Here's how the part is built. I have some questions about the finished solid (model axes, mm). Face numbers are marked on the shaded views. Round coordinates to 2 decimals unless told otherwise and drop trailing zeros. Order: outer loops, then holes, each group sorted by start corner. A loop starts at its lowest first (then second) coordinate and runs counter-clockwise, first axis right, second up.
```python
from build123d import *

# Parameters (mm, degrees)
SKETCH1_W           = 15.24
SKETCH1_H           = 15.24
BOSS_EXTRUDE1_DEPTH = 1.5
SKETCH2_R           = 1.905
SKETCH2_R_2         = 0.635
CUT_EXTRUDE1_DEPTH  = 11.880202204
SKETCH3_W           = 3.95
SKETCH3_H           = 3.95
BOSS_EXTRUDE2_DEPTH = 0.75
BOSS_EXTRUDE3_DEPTH = 0.25


with BuildPart() as part:
    # Sketch1 → Boss-Extrude1 (new body)
    with BuildSketch(Plane(origin=(0, 0, 0), x_dir=(1, 0, 0), z_dir=(0, 1, 0))):
        Rectangle(SKETCH1_W, SKETCH1_H)
    extrude(amount=BOSS_EXTRUDE1_DEPTH)

    # Sketch2 → Cut-Extrude1 (cut, through all)
    with BuildSketch(Plane(origin=(0, 1.5, 0), x_dir=(1, 0, 0), z_dir=(0, 1, 0))):
        with Locations(Location((-5.08, 5.08, 0), (0, 0, 270))):
            Circle(SKETCH2_R)
        with Locations(Location((5.08, 5.08, 0), (0, 0, 270))):
            Circle(SKETCH2_R)
        with Locations(Location((5.08, -6.35, 0), (0, 0, 270))):
            Circle(SKETCH2_R_2)
        with Locations(Location((2.54, -6.35, 0), (0, 0, 270))):
            Circle(SKETCH2_R_2)
        with Locations(Location((0, -6.35, 0), (0, 0, 270))):
            Circle(SKETCH2_R_2)
        with Locations(Location((-2.54, -6.35, 0), (0, 0, 270))):
            Circle(SKETCH2_R_2)
        with Locations(Location((-5.08, -6.35, 0), (0, 0, 270))):
            Circle(SKETCH2_R_2)
    extrude(amount=-CUT_EXTRUDE1_DEPTH, mode=Mode.SUBTRACT)

    # Sketch3 → Boss-Extrude2 (add)
    with BuildSketch(Plane(origin=(0, 1.5, 0), x_dir=(1, 0, 0), z_dir=(0, 1, 0))):
        Rectangle(SKETCH3_W, SKETCH3_H)
    extrude(amount=BOSS_EXTRUDE2_DEPTH)

    # Sketch4 → Boss-Extrude3 (add)
    with BuildSketch(Plane(origin=(0, 2.25, 0), x_dir=(1, 0, 0), z_dir=(0, 1, 0))):
        with BuildLine():
            Line((-1.295144256, 1.380499313), (-1.087590503, 1.380499313))
            add(Edge.make_bspline(
                [(-1.087590503, 1.380499313), (-1.073314825, 1.38048362), (-1.04596199, 1.380453553), (-1.006738628, 1.379541951), (-0.971115209, 1.378324356), (-0.939168546, 1.376636498), (-0.910800345, 1.374641815), (-0.886138971, 1.371844174), (-0.864990582, 1.368923085), (-0.85231887, 1.365953279), (-0.846539822, 1.364598872)],
                knots=[0, 0, 0, 0, 1.415646017, 2.712440637, 3.8905458, 4.950247383, 5.884950622, 6.709939814, 7.411656543, 8, 8, 8, 8], degree=3))
            add(Edge.make_bspline(
                [(-0.846539822, 1.364598872), (-0.839224159, 1.362596521), (-0.824765215, 1.358639001), (-0.803930852, 1.35071247), (-0.784108618, 1.341313815), (-0.765230504, 1.33060229), (-0.747528493, 1.318118322), (-0.730738476, 1.304367966), (-0.715008625, 1.289033754), (-0.700427395, 1.272287673), (-0.687036515, 1.254410848), (-0.675506825, 1.235136412), (-0.66585264, 1.214788803), (-0.65757246, 1.193382176), (-0.651612999, 1.170736768), (-0.64712358, 1.147009929), (-0.644274054, 1.122204201), (-0.644001137, 1.105252765), (-0.643862205, 1.096623445)],
                knots=[0, 0, 0, 0, 0.999701418, 1.975846123, 2.934577507, 3.890451536, 4.834027766, 5.787354733, 6.749476667, 7.726910423, 8.712836071, 9.690891519, 10.682875813, 11.679750201, 12.712814741, 13.765529915, 14.8625177, 16, 16, 16, 16], degree=3))
            add(Edge.make_bspline(
                [(-0.643862205, 1.096623445), (-0.643989636, 1.087921593), (-0.644238963, 1.070895833), (-0.647231411, 1.045987871), (-0.651262207, 1.022184929), (-0.657460125, 0.999539786), (-0.665577745, 0.978186922), (-0.675100342, 0.957800025), (-0.686585838, 0.938725934), (-0.699783203, 0.920895401), (-0.714464281, 0.904291689), (-0.730566955, 0.889035121), (-0.748026217, 0.875214999), (-0.766786581, 0.862800343), (-0.78703094, 0.852079039), (-0.808452258, 0.842476235), (-0.831236728, 0.834411414), (-0.847003631, 0.830168991), (-0.855020057, 0.828012)],
                knots=[0, 0, 0, 0, 1.121902311, 2.195077645, 3.232258892, 4.234102512, 5.217864754, 6.176164875, 7.132989551, 8.084763148, 9.034132444, 9.988522005, 10.94243251, 11.903244335, 12.886203696, 13.894208494, 14.929344452, 16, 16, 16, 16], degree=3))
            add(Edge.make_bspline(
                [(-0.855020057, 0.828012), (-0.861650466, 0.826602003), (-0.87618139, 0.823511913), (-0.900112642, 0.820062213), (-0.927975652, 0.817117748), (-0.959732389, 0.814910024), (-0.995354348, 0.813020031), (-1.0348608, 0.811517774), (-1.078329294, 0.810692318), (-1.108649409, 0.810649745), (-1.124479526, 0.810627518)],
                knots=[0, 0, 0, 0, 0.601384939, 1.31797006, 2.144135048, 3.087295005, 4.142315834, 5.309527816, 6.595305764, 8, 8, 8, 8], degree=3))
            Line((-1.124479526, 0.810627518), (-1.200165624, 0.810627518))
            Line((-1.200165624, 0.810627518), (-1.200165624, 0.322165979))
            Line((-1.200165624, 0.322165979), (-1.295144256, 0.322165979))
            Line((-1.295144256, 0.322165979), (-1.295144256, 1.380499313))
        make_face()
        with BuildLine():
            Line((-1.200165624, 1.271952304), (-1.200165624, 0.919174527))
            Line((-1.200165624, 0.919174527), (-1.014872488, 0.916842462))
            add(Edge.make_bspline(
                [(-1.014872488, 0.916842462), (-1.005825272, 0.916837786), (-0.988359809, 0.916828759), (-0.963130284, 0.918033815), (-0.93972319, 0.919424928), (-0.918210426, 0.921461743), (-0.898582293, 0.92434079), (-0.880806064, 0.927247197), (-0.865019576, 0.931451913), (-0.846544342, 0.937113413), (-0.825957234, 0.946769228), (-0.803560618, 0.960784552), (-0.784579989, 0.978649432), (-0.76815517, 0.998735943), (-0.755120774, 1.021081632), (-0.745578843, 1.044990573), (-0.73997235, 1.070217565), (-0.739220572, 1.087479931), (-0.738840837, 1.096199433)],
                knots=[0, 0, 0, 0, 1.160613943, 2.240541288, 3.23993089, 4.169200891, 5.011653406, 5.7853311, 6.478053781, 7.106038997, 8.262395093, 9.384106736, 10.481365981, 11.59014053, 12.70357646, 13.786202915, 14.881775077, 16, 16, 16, 16], degree=3))
            add(Edge.make_bspline(
                [(-0.738840837, 1.096199433), (-0.739222638, 1.104707984), (-0.739981609, 1.121621929), (-0.745622787, 1.146410745), (-0.755102222, 1.170067731), (-0.768242669, 1.192133402), (-0.784190582, 1.212147636), (-0.802726336, 1.229533672), (-0.823806298, 1.243510235), (-0.843415168, 1.252531251), (-0.860832669, 1.258039203), (-0.875961381, 1.261893), (-0.893043085, 1.264969909), (-0.912083342, 1.267461378), (-0.932934575, 1.26959421), (-0.955775923, 1.271041399), (-0.980520858, 1.271888506), (-0.997699292, 1.271930523), (-1.006604259, 1.271952304)],
                knots=[0, 0, 0, 0, 1.120700087, 2.227813068, 3.331159281, 4.466773991, 5.599788987, 6.693661531, 7.80175334, 8.91857717, 9.525282508, 10.207424825, 10.974604443, 11.810962634, 12.737642355, 13.736264703, 14.826523623, 16, 16, 16, 16], degree=3))
            Line((-1.006604259, 1.271952304), (-1.200165624, 1.271952304))
        make_face(mode=Mode.SUBTRACT)
    extrude(amount=BOSS_EXTRUDE3_DEPTH)


solid = part.part
```
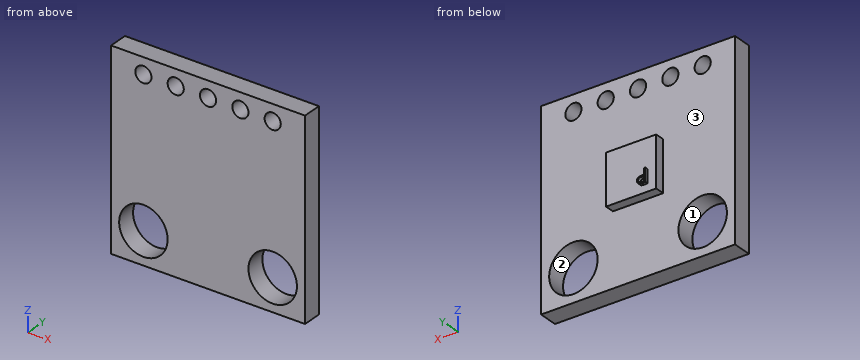
1) I'm going to push flat-ended pins straight in: pin 1 (2 mm diameter, centred on x = -5.08, z = 6.35, fed in from -Y); pin 2 (5 mm diameter, centred on x = -5.08, z = -5.08, fed in from +Y); pin 3 (4.5 mm diameter, centred on x = -3, z = -3, fed in from +Y); pin 4 (0.8 mm diameter, centred on x = 1, y = 2, fed in from +Z) (3 decimals). Where does each tip first touch, or does it pass through?
2) If we section it at D-D (x = -5.08): Write out the boundary of the cut face in (y, z) (3 decimals), plus the area to 3 significant figures.
3) We'd pull the mould along X, two halves only. Please class the marked faces 1, 2 and 3: +X half, -X half, draft (parallel to the pull), parting line (faces both ways), or undercut.
4) If we section it at A-A (x = 0): Write out the boundary of the cut face in (y, z) (3 decimals).
5) I need wall thicknesses on line 1 (X direction, y = 0.7, z = 6.35) (3 decimals); line 2 (X direction, y = 0.65, z = -5.08) (3 decimals); line 3 (Z direction, x = 4.75, y = 0.2). Which ranges of each line are inside material? Lowest first, please.
6) If we section it at C-C (y = 0.75): Write out the boundary of the cut face in (x, z) (3 decimals).
7) If we section it at B-B (z = -5.08): Write out the boundary of the cut face in (x, y) (3 decimals).
Solutions:
1. pin 1: stops at y = 0
1. pin 2: stops at y = 1.5
1. pin 3: stops at y = 2.25
1. pin 4: stops at z = 1.975
2. outline: (0, -7.62) - (1.5, -7.62) - (1.5, -6.985) - (0, -6.985) - close; (0, -3.175) - (1.5, -3.175) - (1.5, 5.715) - (0, 5.715) - close; (0, 6.985) - (1.5, 6.985) - (1.5, 7.62) - (0, 7.62) - close
2. area: 15.2 mm2
3. face 1: undercut
3. face 2: undercut
3. face 3: draft
4. outline: (0, -7.62) - (1.5, -7.62) - (1.5, -1.975) - (2.25, -1.975) - (2.25, 1.975) - (1.5, 1.975) - (1.5, 5.715) - (0, 5.715) - close; (0, 6.985) - (1.5, 6.985) - (1.5, 7.62) - (0, 7.62) - close
5. line 1: x = -7.62 to -5.715, -4.445 to -3.175, -1.905 to -0.635, 0.635 to 1.905, 3.175 to 4.445, 5.715 to 7.62
5. line 2: x = -7.62 to -6.985, -3.175 to 3.175, 6.985 to 7.62
5. line 3: z = -7.62 to -6.96, -3.2 to 5.81, 6.89 to 7.62
6. outline: (-7.62, -7.62) - (7.62, -7.62) - (7.62, 7.62) - (-7.62, 7.62) - close; hole circle Ø3.81 at (-5.08, -5.08); hole circle Ø1.27 at (-5.08, 6.35); hole circle Ø1.27 at (-2.54, 6.35); hole circle Ø1.27 at (0, 6.35); hole circle Ø1.27 at (2.54, 6.35); hole circle Ø3.81 at (5.08, -5.08); hole circle Ø1.27 at (5.08, 6.35)
7. outline: (-7.62, 0) - (-6.985, 0) - (-6.985, 1.5) - (-7.62, 1.5) - close; (-3.175, 0) - (3.175, 0) - (3.175, 1.5) - (-3.175, 1.5) - close; (6.985, 0) - (7.62, 0) - (7.62, 1.5) - (6.985, 1.5) - close
